Read the model definition and answer for the solid it produces. Units are mm, in the model's axes. A direction names the side the tool comes from. Round coordinates to 2 decimals unless told otherwise and drop trailing zeros. Order: outer loops, then holes, each group sorted by start corner. A loop starts at its lowest first (then second) coordinate and runs counter-clockwise, first axis right, second up. Notation, with made-up numbers: (-35.75, 79) -> (-0.75, 79) arc R14 ccw to (-0.75, 104) -> close; hole circle Ø5 at (0.5, 16). An arc over 180 degrees is marked (long way). Use a Markdown table: item, result. Add a question column.
1. Section A-A, the plane z = 0.6 is taken. Give the vertices of the cut face in (x, y).
2. Section C-C, the plane y = -83.5 is taken. Give the vertices of the cut face in (x, z), then the cut area to 3 significant figures.
3. The mould has two halves that part along X. Classify faces 1 (the face through (144.038, -24.295, 1.972)), 2 (the face through (41, -38, 4)), 3 (the face through (70, -7, 2)): +X half, -X half, draft (parallel to the pull), parting line (faces both ways), or undercut.
4. Given pin 1 (1 mm diameter, centred on x = 111.5, z = 2.5, fed in from -Y), flat-ended and moving along its own axis, determine where the tip first touches the part or whether it passes through.
5. For faces 4 (the face through (41, -38, 0)), 5 (the face through (145, -7, 2)), 6 (the face through (120, -29, 2)), determine the directions among +Z, -Z, +X, -X, +Y, -Y from which every point of the face is accessible in a straight line to the end or side of a thin tool.
6. Consider L1, parallel to X at y = -18.5, z = 2.35; L2, parallel to X at y = -60, z = 3.1; L3, parallel to X at y = -43, z = 2.15. Determine where each line is inside the solid, lowest interval first. Write a range as [from, to].
7. Section B-B, the plane x = 22 is taken. Give the vertices of the cut face in (y, z).
```python
from build123d import *

# Parameters (mm, degrees)
F1_DEPTH = 4


with BuildPart() as f1:
    # F0 (on Top) → F1 (new body)
    with BuildSketch(Plane.XY):
        with BuildLine():
            Line((5, 0), (0, -5))
            Line((0, -5), (0, -100))
            Line((0, -100), (27.486404, -85.706576))
            Line((27.486404, -85.706576), (108.429266, -29))
            Line((108.429266, -29), (132.5, -29))
            ThreePointArc((132.5, -29), (144.167262, -24.167262), (149, -12.5))
            Line((149, -12.5), (150, 0))
            Line((150, 0), (145.965368, 0))
            Line((145.965368, 0), (145, -1.158226))
            Line((145, -1.158226), (145, -3.333333))
            Line((145, -3.333333), (145, -12.5))
            ThreePointArc((145, -12.5), (132.5, -25), (120, -12.5))
            Line((120, -12.5), (120, -2))
            Line((120, -2), (118, 0))
            Line((118, 0), (96.858531, 0))
            Line((96.858531, 0), (95, -2))
            Line((95, -2), (95, -12.5))
            ThreePointArc((95, -12.5), (82.5, -25), (70, -12.5))
            Line((70, -12.5), (70, -2))
            Line((70, -2), (68, 0))
            Line((68, 0), (5, 0))
        make_face()
    extrude(amount=F1_DEPTH)


solid = f1.part
```
Verdict:
| question | item | result |
|---|---|---|
| 1 | outline | (0, -100) -> (27.49, -85.71) -> (108.43, -29) -> (132.5, -29) arc R16.5 ccw to (149, -12.5) -> (150, 0) -> (145.97, 0) -> (145, -1.16) -> (145, -12.5) arc R12.5 cw to (120, -12.5) -> (120, -2) -> (118, 0) -> (96.86, 0) -> (95, -2) -> (95, -12.5) arc R12.5 cw to (70, -12.5) -> (70, -2) -> (68, 0) -> (5, 0) -> (0, -5) -> close |
| 2 | outline | (0, 0) -> (30.64, 0) -> (30.64, 4) -> (0, 4) -> close |
| 2 | area | 123 mm2 |
| 3 | face 1 | +X half |
| 3 | face 2 | draft |
| 3 | face 3 | undercut |
| 4 | pin 1 | stops at y = -29 |
| 5 | face 4 | -Z, +X, -X, +Y, -Y |
| 5 | face 5 | +Z, -Z, +Y |
| 5 | face 6 | +Z, -Z, +X, -Y |
| 6 | L1 | x = [0, 71.53], [93.47, 121.53], [143.47, 147.87] |
| 6 | L2 | x = [0, 64.18] |
| 6 | L3 | x = [0, 88.45] |
| 7 | outline | (-88.56, 0) -> (0, 0) -> (0, 4) -> (-88.56, 4) -> close |
